```python
from build123d import *

# Parameters (mm, degrees)
BOSS_EXTRUDE1_DEPTH = 15
SKETCH3_W           = 32.23682377
SKETCH3_H           = 8.180060941
BOSS_EXTRUDE2_DEPTH = 15
SKETCH4_R           = 1
CUT_EXTRUDE1_DEPTH  = 15


with BuildPart() as part:
    # Sketch2 → Boss-Extrude1 (new body)
    with BuildSketch(Plane(origin=(0, 0, 0), x_dir=(1, 0, 0), z_dir=(0, 1, 0))):
        with BuildLine():
            Line((-16.118411885, 13.460936011), (-15.350868462, 12.819939059))
            ThreePointArc((-15.350868462, 12.819939059), (0, 20), (15.350868462, 12.819939059))
            Line((15.350868462, 12.819939059), (16.118411885, 13.460936011))
            ThreePointArc((16.118411885, 13.460936011), (0, 21), (-16.118411885, 13.460936011))
        make_face()
    extrude(amount=BOSS_EXTRUDE1_DEPTH)

    # Sketch3 → Boss-Extrude2 (add)
    with BuildSketch(Plane.XZ):
        with Locations((0, -16.909969529)):
            Rectangle(SKETCH3_W, SKETCH3_H)
    extrude(amount=BOSS_EXTRUDE2_DEPTH)

    # Sketch4 → Cut-Extrude1 (cut)
    with BuildSketch(Plane(origin=(16.118411885, 0, 0), x_dir=(0, 0, -1), z_dir=(1, 0, 0))):
        with Locations((16.909969529, -12.5)):
            Circle(SKETCH4_R)
        with Locations((16.909969529, -8.5)):
            Circle(SKETCH4_R)
    extrude(amount=-CUT_EXTRUDE1_DEPTH, mode=Mode.SUBTRACT)


solid = part.part
```
Verification items for the finished model (mm, model axes). A direction names the side the tool comes from. Round coordinates to 2 decimals unless told otherwise and drop trailing zeros. Write each loop counter-clockwise with the first axis right and the second up, starting at its lowest first coordinate (ties: lowest second). Pieces come first, ordered by that corner, then holes.
1. Draft check along Z on faces 4 (the flat face through (1.118, -12, -17)), 5 (the flat face through (-0.1, 15, -20.3)), 6 (the cylindrical face through (0, 7, -21)). Enter one of: +Z half, -Z half, draft (parallel to the pull), parting line (faces both ways), or undercut.
2. Section check B-B on y = -12.5. Enter the section's corners in (x, z).
3. Section check A-A on x = 6. Enter the section's corners in (y, z), plus the area to 3 significant figures.
4. Gauge pin test, flat ends, axial feed: P1, Ø1.5, axis at x = -1.5, y = 7, coming from the -Z side; P2, Ø2, axis at y = 10, z = -19, coming from the +X side. Record the tip position at first contact, or that the pin passes through.
5. Section check C-C on z = -20.5. Enter the section's corners in (x, y).
6. Scan lines: L1, parallel to Y at x = -6.5, z = -16.75; L2, parallel to X at y = 12.25, z = -15.75; L3, parallel to X at y = 11, z = -14.5. Record each from-to range of solid material in increasing order.
7. Access from +Z, -Z, +X, -X, +Y, -Y to the whole of each face (thin tool, end or side, straight path). Record for faces 1 (the flat face through (12, 0, -19)), 2 (the cylindrical face through (0, 7, -20)), 3 (the cylindrical face through (8.72, -7.66, -17.45)).
8. Section check D-D on z = -18.75. Enter the section's corners in (x, y).
Answer:
1. face 4: undercut
1. face 5: draft
1. face 6: -Z half
2. outline: (-16.12, -21) - (16.12, -21) - (16.12, -17.91) - (1.12, -17.91) - (1.12, -15.91) - (16.12, -15.91) - (16.12, -12.82) - (-16.12, -12.82) - close
3. outline: (-15, -21) - (0, -21) - (0, -20.12) - (15, -20.12) - (15, -19.08) - (0, -19.08) - (0, -12.82) - (-15, -12.82) - close; hole circle Ø2 at (-12.5, -16.91); hole circle Ø2 at (-8.5, -16.91)
3. area: 132 mm2
4. P1: stops at z = -20.99
4. P2: stops at x = 10.82
5. outline: (-16.12, -15) - (16.12, -15) - (16.12, 0) - (4.56, 0) - (4.56, 15) - (-4.56, 15) - (-4.56, 0) - (-16.12, 0) - close
6. L1: y = -15 to 0
6. L2: x = -13.89 to -12.33, 12.33 to 13.89
6. L3: x = -15.19 to -13.77, 13.77 to 15.19
7. face 1: -Z, +X, +Y
7. face 2: +Z, +Y
7. face 3: +X
8. outline: (-16.12, -15) - (16.12, -15) - (16.12, 0) - (9.46, 0) - (9.46, 15) - (6.96, 15) - (6.96, 0) - (-6.96, 0) - (-6.96, 15) - (-9.46, 15) - (-9.46, 0) - (-16.12, 0) - close
